```python
from build123d import *

# Parameters (mm, degrees)
SKETCH1_R               = 7.975
BOSS_EXTRUDE1_DEPTH     = 44
SKETCH2_R               = 1.5
CUT_EXTRUDE1_DEPTH      = 46.422475164
LPATTERN3_PLANET2_COUNT = 4
LPATTERN3_PLANET2_PITCH = 3.001


with BuildPart() as part:
    # Sketch1 → Boss-Extrude1 (new, symmetric)
    with BuildSketch(Plane.XY):
        Circle(SKETCH1_R)
    extrude(amount=BOSS_EXTRUDE1_DEPTH, both=True)

    # Sketch2 → Cut-Extrude1 (cut, symmetric)
    with BuildSketch(Plane(origin=(0, 0, 0), x_dir=(1, 0, 0), z_dir=(0, 1, 0))):
        with Locations(Location((0, -39.5, 0), (0, 0, 270))):
            Circle(SKETCH2_R)
    cut_extrude1 = extrude(amount=CUT_EXTRUDE1_DEPTH, both=True, mode=Mode.SUBTRACT)

    # LPattern3-Planet2: Cut-Extrude1 ×4
    with Locations(*[(0, 0, -i * LPATTERN3_PLANET2_PITCH) for i in range(1, LPATTERN3_PLANET2_COUNT)]):
        add(cut_extrude1, mode=Mode.SUBTRACT)


solid = part.part
```
Here's how the part is built. I have some questions about the finished solid (model axes, mm). Coordinates: 2 decimals unless noted, no trailing zeros. Write each loop counter-clockwise with the first axis right and the second up, starting at its lowest first coordinate (ties: lowest second). Pieces come first, ordered by that corner, then holes. Notation, with made-up numbers: (-12.75, -40) - (8.25, -40) arc R17 ccw to (8.25, -14) - close; hole circle Ø9 at (-1.75, -14.5). An arc over 180 degrees is marked (long way). One line per item, written item: value.
1) Suppose I cut it at A-A on x = 0. State how many separate pieces and enclosed holes the cut face has, and give its area (3 significant figures).
Model answer:
separate pieces: 5
enclosed holes: 0
area: 1,210 mm²
2) Suppose I cut it at D-D on y = -3.25. Write out the boundary of the cut face in (x, z), and give its area (3 significant figures).
Model answer:
outline: (-7.28, -44) - (7.28, -44) - (7.28, 44) - (-7.28, 44) - close; hole circle Ø3 at (0, 30.5); hole circle Ø3 at (0, 33.5); hole circle Ø3 at (0, 36.5); hole circle Ø3 at (0, 39.5)
area: 1,250 mm²
3) Suppose I cut it at C-C on z = 39.5. Write out the boundary of the cut face in (x, y) (3 decimals).
Model answer:
outline: (-1.5, -7.833) - (-1.5, 7.833) arc R7.975 ccw to start; (1.5, -7.833) arc R7.975 ccw to (1.5, 7.833) - close
4) We'd pull the mould along Z, two halves only. Please class faces 1 (the flat face through (0, 0, 44)), 2 (the flat face through (0, 0, -44)), 3 (the cylindrical face through (-0.9, 0.1, 35.3)): pulls with the +Z half, pulls with the -Z half, needs draft (parallel to the pull), parting line crosses it, or undercut.
Model answer:
face 1: pulls with the +Z half
face 2: pulls with the -Z half
face 3: undercut
5) Suppose I cut it at B-B on y = 0. Write out the boundary of the cut face in (x, z) (3 decimals).
Model answer:
outline: (-7.975, -44) - (7.975, -44) - (7.975, 44) - (-7.975, 44) - close; hole circle Ø3 at (0, 30.497); hole circle Ø3 at (0, 33.498); hole circle Ø3 at (0, 36.499); hole circle Ø3 at (0, 39.5)
6) I'm going to push flat-ended pins straight in: P1, Ø4, axis at x = -2, z = 11.5, coming from the +Y side (3 decimals); P2, Ø1.8, axis at x = 0, z = 39.5, coming from the +Y side; P3, Ø3, axis at y = -3, z = -4.5, coming from the -X side. Where does each tip first touch, or does it pass through?
Model answer:
P1: stops at y = 7.975
P2: passes through
P3: stops at x = -7.83
7) I need wall thicknesses on line 1 along Z through (x, y) = (1.25, 3); line 2 along Z through (x, y) = (-1, -4.75); line 3 along X through (y, z) = (-4.25, 39.5). Which ranges of each line are inside material? Lowest first, please.
Model answer:
line 1: z = -44 to 29.67, 31.33 to 32.67, 34.33 to 35.67, 37.33 to 38.67, 40.33 to 44
line 2: z = -44 to 29.38, 31.62 to 32.38, 34.62 to 35.38, 37.62 to 38.38, 40.62 to 44
line 3: x = -6.75 to -1.5, 1.5 to 6.75
